Can you work these out from the model? Positions are in its coordinate system, mm. A direction names the side the tool comes from. Round coordinates to 2 decimals unless told otherwise and drop trailing zeros. Loops run counter-clockwise (first coordinate to the right, second up) from the corner with the lowest first, then second, coordinate; pieces in that order, holes last.
from build123d import *

# Parameters (mm, degrees)
BOSS_EXTRUDE1_DEPTH = 10
BOSS_EXTRUDE3_DEPTH = 5
FILLET1_R           = 5
SKETCH5_R           = 1.65
CUT_EXTRUDE2_DEPTH  = 20
CHAMFER1_SIZE       = 1


with BuildPart() as part:
    # Sketch1 → Boss-Extrude1 (new body)
    with BuildSketch(Plane(origin=(0, 0, 0), x_dir=(1, 0, 0), z_dir=(0, 1, 0))):
        with BuildLine():
            Line((0, 33), (35, 33))
            Line((35, 33), (35, 13))
            Line((35, 13), (0, 13))
            ThreePointArc((0, 13), (-13, 0), (0, -13))
            Line((0, -13), (35, -13))
            Line((35, -13), (35, -33))
            Line((35, -33), (0, -33))
            ThreePointArc((0, -33), (-33, 0), (0, 33))
        make_face()
    extrude(amount=BOSS_EXTRUDE1_DEPTH)

    # Sketch4 → Boss-Extrude3 (add)
    with BuildSketch(Plane(origin=(0, 10, 0), x_dir=(1, 0, 0), z_dir=(0, 1, 0))):
        with BuildLine():
            Line((0, 15), (35, 15))
            Line((35, 15), (35, 33))
            Line((35, 33), (0, 33))
            ThreePointArc((0, 33), (-33, 0), (0, -33))
            Line((0, -33), (35, -33))
            Line((35, -33), (35, -15))
            Line((35, -15), (0, -15))
            ThreePointArc((0, -15), (-15, 0), (0, 15))
        make_face()
    extrude(amount=BOSS_EXTRUDE3_DEPTH)

    # Fillet1
    fillet1_edges = [part.edges().sort_by_distance(p)[0] for p in [
        (35, 7.5, -33),
        (35, 5, -13),
        (35, 5, 13),
        (35, 7.5, 33),
    ]]
    fillet(fillet1_edges, radius=FILLET1_R)

    # Sketch5 → Cut-Extrude2 (cut)
    with BuildSketch(Plane(origin=(0, 15, 0), x_dir=(1, 0, 0), z_dir=(0, 1, 0))):
        with Locations((25, 23)):
            Circle(SKETCH5_R)
        with Locations((25, -23)):
            Circle(SKETCH5_R)
    extrude(amount=-CUT_EXTRUDE2_DEPTH, mode=Mode.SUBTRACT)

    # Chamfer1
    chamfer1_edges = [part.edges().sort_by_distance(p)[0] for p in [
        (15, 0, 33),
        (-33, 0, 0),
        (-15, 15, 0),
        (17, 15, -15),
        (-33, 15, 0),
        (15, 15, 33),
        (15, 0, -33),
        (15, 15, -33),
        (35, 0, -23),
        (15, 0, 13),
        (35, 0, 23),
        (33.535533906, 0, 31.535533906),
        (33.535533906, 0, 14.464466094),
        (33.535533906, 0, -14.464466094),
        (33.535533906, 0, -31.535533906),
        (35, 15, -23),
        (35, 15, 23),
        (17, 15, 15),
        (33.535533906, 15, 31.535533906),
        (34.74341649, 15, 16.41886117),
        (34.74341649, 15, -16.41886117),
        (33.535533906, 15, -31.535533906),
        (23.35, 0, -23),
        (23.35, 15, -23),
        (23.35, 0, 23),
        (23.35, 15, 23),
        (15, 0, -13),
        (-13, 0, 0),
    ]]
    chamfer(chamfer1_edges, length=CHAMFER1_SIZE)


solid = part.part
(1) For faces 1 (the cylindrical face through (-15, 12, 0)), 2 (the conical face through (33.063, 14.715, -30.996)), 3 (the flat face through (15, 5, 13)), which set-ups out of +Z, -Z, +X, -X, +Y, -Y let a thin tool reach every point of the face, with its end or its side?
Worked answers:
face 1: +X, +Y
face 2: -Z, +X, +Y
face 3: +X, +Y, -Y
(2) If we section it at B-B, the plane x = 9: List the corners of the cut face in (y, z) for me, then the cut area to 3 significant figures.
Worked answers:
outline: (0, -32) - (1, -33) - (14, -33) - (15, -32) - (15, -16) - (14, -15) - (10, -15) - (10, -13) - (1, -13) - (0, -14) - close; (0, 14) - (1, 13) - (10, 13) - (10, 15) - (14, 15) - (15, 16) - (15, 32) - (14, 33) - (1, 33) - (0, 32) - close
area: 576 mm2
(3) If we section it at D-D, the plane x = 25: State how many separate pieces and enclosed holes the cut face has, then the cut area to 3 significant figures.
Worked answers:
separate pieces: 4
enclosed holes: 0
area: 473 mm2
(4) If I drill on line 1 (Z direction, x = 25, y = 7.75); line 2 (Z direction, x = 23, y = 10.25); line 3 (Z direction, x = 17.5, y = 2.5), over which ranges is the centre line in solid material (lowest first)?
Worked answers:
line 1: z = -33 to -24.65, -21.35 to -13, 13 to 21.35, 24.65 to 33
line 2: z = -33 to -15, 15 to 33
line 3: z = -33 to -13, 13 to 33
(5) Will these pins go through, and if not, where does the flat tip stop? P1, Ø6, axis at x = -8.5, z = -7.5, coming from the +Y side; P2, Ø4.5, axis at x = 25, z = -23, coming from the +Y side; P3, Ø6, axis at x = -9.5, y = 12.5, coming from the -Z side.
Worked answers:
P1: stops at y = 10
P2: stops at y = 14.6
P3: stops at z = -32.35
(6) If we section it at C-C, the plane z = 0: List the corners of the cut face in (x, y) for me, then the cut area to 3 significant figures.
Worked answers:
outline: (-33, 1) - (-32, 0) - (-14, 0) - (-13, 1) - (-13, 10) - (-15, 10) - (-15, 14) - (-16, 15) - (-32, 15) - (-33, 14) - close
area: 288 mm2
(7) If we mould it in two halves opening along Z, with no side actions, what happens to faces 4 (the flat face through (35, 7, 23)), 5 (the conical face through (34.282, 14.493, 16.594)), 6 (the conical face through (-32.166, 14.826, -0.707))? For each: released by +Z, released by -Z, zero draft, split by the parting line, or undercut.
Worked answers:
face 4: zero draft
face 5: undercut
face 6: split by the parting line
(8) If we section it at A-A, the plane y = 6: List the corners of the cut face in (x, z) for me.
Worked answers:
outline: (0, -33) - (30, -33) arc R5 ccw to (35, -28) - (35, -18) arc R5 ccw to (30, -13) - (0, -13) arc R13 cw to (0, 13) - (30, 13) arc R5 ccw to (35, 18) - (35, 28) arc R5 ccw to (30, 33) - (0, 33) arc R33 ccw to start; hole circle Ø3.3 at (25, -23); hole circle Ø3.3 at (25, 23)
